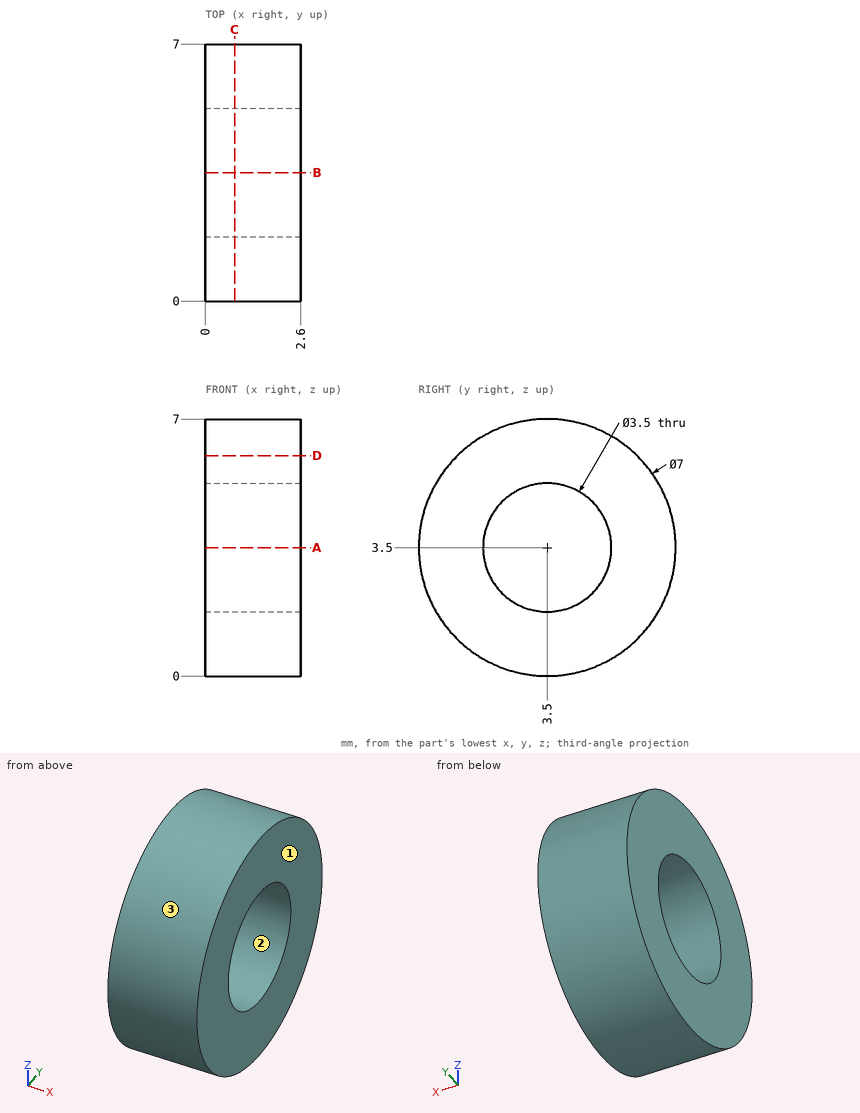
Geometry check sheet. Reference: drawing and pictorial views, mm from the part's lowest x, y, z. Coordinates: 2 decimals unless noted, no trailing zeros. Order: outer loops, then holes, each group sorted by start corner. A loop starts at its lowest first (then second) coordinate and runs counter-clockwise, first axis right, second up. Notation, with made-up numbers: (43.25, 54.25) - (68.25, 54.25) arc R31 cw to (68.25, 79.25) - close; hole circle Ø8 at (-29.75, -6.75). An arc over 180 degrees is marked (long way). One line per item, written item: value.
(1) Release check for a two-part mould opening along Y. For the marked faces 1, 2 and 3 record: +Y half, -Y half, draft (parallel to the pull), parting line (faces both ways), or undercut.
Data:
face 1: draft
face 2: undercut
face 3: parting line
(2) Thickness scan on probe 1 along Z at (x, y) = (0.7, 3.5); probe 2 along Z at (x, y) = (1.4, 2). Record the ranges inside material, lowest first. Write a range as from..to.
Data:
probe 1: z = 0..1.75, 5.25..7
probe 2: z = 0.34..2.6, 4.4..6.66
(3) Depth check by flat-ended pin: pin 1 Ø3 at (y, z) = (3.5, 3.5) entering from -X; pin 2 Ø1 at (x, z) = (2, 0.5) entering from -Y. Enter the tip coordinate at first touch or a pass-through.
Data:
pin 1: passes through
pin 2: stops at y = 1.05
(4) Sectioned sample at C-C (x = 0.8). Enter the section's corners in (y, z), and give its area (3 significant figures).
Data:
outline: circle Ø7 at (3.5, 3.5); hole circle Ø3.5 at (3.5, 3.5)
area: 28.9 mm^2
(5) Sectioned sample at D-D (z = 6). Enter the section's corners in (x, y).
Data:
outline: (0, 1.05) - (2.6, 1.05) - (2.6, 5.95) - (0, 5.95) - close
(6) Sectioned sample at A-A (z = 3.5). Enter the section's corners in (x, y).
Data:
outline: (0, 0) - (2.6, 0) - (2.6, 1.75) - (0, 1.75) - close; (0, 5.25) - (2.6, 5.25) - (2.6, 7) - (0, 7) - close
